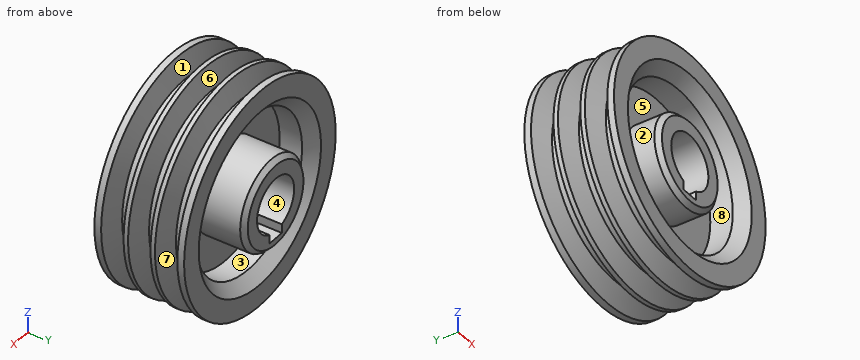
Autodesk Inventor part; units mm, degrees
ref_plane "YZ Plane" through (0, 0, 0) normal (1, 0, 0) x (0, 1, 0)
ref_plane "XZ Plane" through (0, 0, 0) normal (0, 1, 0) x (-1, 0, 0)
ref_plane "XY Plane" through (0, 0, 0) normal (0, 0, 1) x (1, 0, 0)
sketch "Sketch1" plane through (0, 0, 0) normal (0, 0, 1) x (1, 0, 0)
  line L0 (0, 0) -> (0, 47)
  line L1 (0, 0) -> (18, 0)
  line L2 (20, 2) -> (20, 15)
  line L3 (20, 15) -> (35, 15)
  line L4 (35, 15) -> (35, 5)
  line L5 (40, 0) -> (49, 0)
  line L6 (49, 0) -> (49, 3)
  line L7 (49, 3) -> (39.7669, 6)
  line L8 (39.7669, 6) -> (39.7669, 10)
  line L9 (39.7669, 10) -> (49, 13)
  line L10 (49, 13) -> (49, 15)
  line L11 (49, 15) -> (39.7669, 18)
  line L12 (39.7669, 18) -> (39.7669, 22)
  line L13 (39.7669, 22) -> (49, 25)
  line L14 (49, 25) -> (49, 27)
  line L15 (49, 27) -> (39.7669, 30)
  line L16 (39.7669, 30) -> (39.7669, 34)
  line L17 (39.7669, 34) -> (49, 37)
  line L18 (49, 37) -> (49, 40)
  line L19 (49, 40) -> (39.5, 40)
  line L20 (34.5, 35) -> (34.5, 25)
  line L21 (34.5, 25) -> (20, 25)
  line L22 (20, 25) -> (20, 45)
  line L23 (18, 47) -> (0, 47)
  line L24 (18, 47) -> (20, 45)
  line L25 (20, 2) -> (18, 0)
  line L26 (35, 5) -> (40, 0)
  line L27 (34.5, 35) -> (39.5, 40)
  point P0 (20, 0)
  point P1 (35, 0)
  point P2 (39.7669, 8)
  point P3 (39.7669, 20)
  point P4 (34.5, 40)
  point P5 (20, 47)
  dimension "d0" = 40
  dimension "d1" = 70
  dimension "d2" = 98
  dimension "d3" = 15
  dimension "d4" = 4
  dimension "d5" = 10
  dimension "d6" = 8
  dimension "d7" = 12
  dimension "d8" = 36
  dimension "d9" = 18
  dimension "d10" = 40
  dimension "d11" = 15
  dimension "d12" = 40
  dimension "d13" = 47
  dimension "d14" = 2
  dimension "d15" = 45
  dimension "d16" = 2
  dimension "d17" = 45
  dimension "d18" = 5
  dimension "d19" = 45
  dimension "d20" = 5
  dimension "d21" = 45
  dimension "d22" = 9.5
revolve "Revolution1" add sketch "Sketch1" angle 360 about axis through (0, 0, 0) along (0, 1, 0)
sketch "Sketch2" plane through (0, 47, 0) normal (0, 1, 0) x (1, 0, 0)
  circle A0 centre (0, 0) radius 12
  line L0 (-4, 11.3137) -> (-4, 15.3)
  line L1 (-4, 15.3) -> (4, 15.3)
  line L2 (4, 15.3) -> (4, 11.3137)
  point P0 (0, -12)
  dimension "d24" = 24
  dimension "d25" = 27.3
  dimension "d26" = 8
extrude "Extrusion1" cut sketch "Sketch2" against normal up to surface (47 mm away)
equation "\"d9\" = 0.5 * d8"
equation "\"d17\" = d15"
equation "\"d21\" = d19"
properties part number "V-Belt_Pulley_3_Groove"
Geometry: final body of the model. Coordinates: model frame, mm. Face numbers are marked on the shaded views. A direction names the side the tool comes from. Give positions to 0.01 mm unless a question says otherwise; leave off trailing zeros. Return JSON: item names as keys, results as strings.
Item 1: Pin query (flat end, axial travel): P1, Ø14.5, axis at x = 0, z = 0, coming from the -Y side; P2, Ø4, axis at x = 35, z = 28, coming from the -Y side; P3, Ø2, axis at x = 4, z = 31.5, coming from the -Y side; P4, Ø2, axis at y = 15, z = -13, coming from the -X side. Return the tip coordinate at first contact, or that it passes through.
Filled in:
{"P1": "through", "P2": "y = 0", "P3": "y = 15", "P4": "x = -47.51"}
Item 2: Line query: line 1 (X direction, y = 32, z = 0); line 2 (Z direction, x = 0, y = 30.5); line 3 (X direction, y = 26, z = 0). Output: solid intervals per line, ascending.
Filled in:
{"line 1": "-39.77 to -34.5, -20 to -12, 12 to 20, 34.5 to 39.77", "line 2": "-39.77 to -34.5, -20 to -15.3, 12 to 20, 34.5 to 39.77", "line 3": "-49 to -34.5, -20 to -12, 12 to 20, 34.5 to 49"}
Item 3: Mould query, pull axis Y, two halves, no side actions, for the marked faces 5, 6, 7 and 8. Classes: released by +Y, released by -Y, zero draft, split by the parting line, or undercut.
Filled in:
{"face 5": "released by -Y", "face 6": "undercut", "face 7": "undercut", "face 8": "zero draft"}
Item 4: Access query for the marked faces 1, 2, 3 and 4. Directions: +Z, -Z, +X, -X, +Y, -Y. A direction counts if a zero-diameter tool reaches every point of the face in a straight line with its end or side. Return the directions, or none.
Filled in:
{"face 1": "none", "face 2": "-Y", "face 3": "+Y", "face 4": "+Y, -Y"}
